Geometry: final body of the model. Coordinates: model frame, mm. Face numbers are marked on the shaded views. Round coordinates to 2 decimals unless told otherwise and drop trailing zeros. Loops run counter-clockwise (first coordinate to the right, second up) from the corner with the lowest first, then second, coordinate; pieces in that order, holes last. Notation, with made-up numbers: (-4, 67.25) - (54, 67.25) arc R18 ccw to (54, 100.25) - close; hole circle Ø6 at (-18, 29.25). An arc over 180 degrees is marked (long way). Return JSON: item names as keys, results as strings. Group by question number.
1. Section C-C on z = 154. Return loops of the section in (x, y), and give its area (3 significant figures).
2. Draft query along X for the marked faces 1 and 2. Return one class per face: +X half, -X half, draft (parallel to the pull), parting line (faces both ways), or undercut.
3. Section D-D on x = 34.5. Return loops of the section in (y, z).
4. Material intervals for probe 1 along Z at (x, y) = (88.9, -0.6); probe 2 along Z at (x, y) = (60, -0.1); probe 3 along Z at (x, y) = (94.5, -0.65), sorted ascending.
5. First-contact query: pin 1 Ø3 at (x, z) = (51.5, 147) entering from +Y. Flat tip, straight axial feed; report the tip coordinate or a pass-through.
6. Section A-A on y = -0.2. Return loops of the section in (x, z).
7. Section B-B on x = 88.9. Return loops of the section in (y, z).
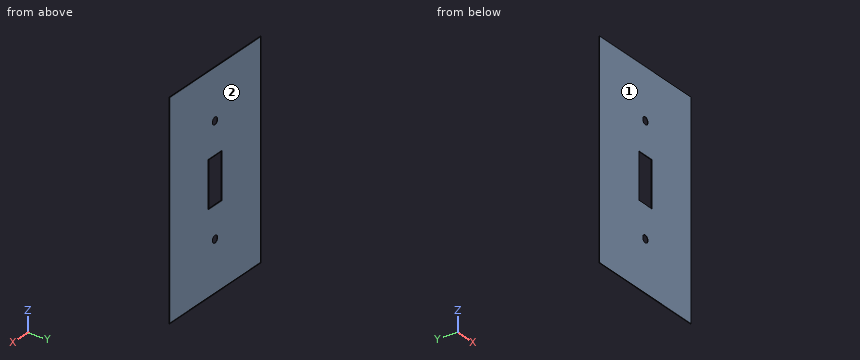
from build123d import *

# Parameters (mm, degrees)
F0_W     = 177.8
F0_H     = 292.1
F1_DEPTH = 1.016
F3_W     = 25.4
F3_H     = 63.5
F4_DEPTH = 25.4
F5_T     = -0.508
F6_R     = 5.08
F7_DEPTH = 25.4
F8_R     = 5.08
F9_DEPTH = 25.4


with BuildPart() as f1:
    # F0 (on Front) → F1 (new body)
    with BuildSketch(Plane.XZ):
        with Locations((88.9, 146.05)):
            Rectangle(F0_W, F0_H)
    extrude(amount=F1_DEPTH)

    # F3 (on face) → F4 (cut)
    with BuildSketch(Plane.XZ.offset(1.016)):
        with Locations((88.9, 146.05)):
            Rectangle(F3_W, F3_H)
    extrude(amount=-F4_DEPTH, mode=Mode.SUBTRACT)

    # F5
    f5_openings = [f1.faces().sort_by_distance(p)[0] for p in [
        (3.41958, 0, 146.05),
    ]]
    offset(amount=F5_T, openings=f5_openings, kind=Kind.INTERSECTION)

    # F6 (on face) → F7 (cut)
    with BuildSketch(Plane.XZ.offset(1.016)):
        with Locations((88.9, 69.85)):
            Circle(F6_R)
    extrude(amount=-F7_DEPTH, mode=Mode.SUBTRACT)

    # F8 (on face) → F9 (cut)
    with BuildSketch(Plane.XZ.offset(1.016)):
        with Locations((88.9, 222.25)):
            Circle(F8_R)
    extrude(amount=-F9_DEPTH, mode=Mode.SUBTRACT)


solid = f1.part
Taken from the geometry:
{
 "1": {"outline": "(0, -1.02) - (76.2, -1.02) - (76.2, 0) - (75.69, 0) - (75.69, -0.51) - (0.51, -0.51) - (0.51, 0) - (0, 0) - close; (101.6, -1.02) - (177.8, -1.02) - (177.8, 0) - (177.29, 0) - (177.29, -0.51) - (102.11, -0.51) - (102.11, 0) - (101.6, 0) - close", "area": "78.5 mm2"},
 "2": {"face 1": "draft", "face 2": "undercut"},
 "3": {"outline": "(-1.02, 0) - (0, 0) - (0, 0.51) - (-0.51, 0.51) - (-0.51, 291.59) - (0, 291.59) - (0, 292.1) - (-1.02, 292.1) - close"},
 "4": {"probe 1": "0 to 64.77, 74.93 to 114.3, 177.8 to 217.17, 227.33 to 292.1", "probe 2": "0 to 0.51, 291.59 to 292.1", "probe 3": "0 to 114.3, 177.8 to 292.1"},
 "5": {"pin 1": "y = -0.51"},
 "6": {"outline": "(0, 0) - (177.8, 0) - (177.8, 292.1) - (0, 292.1) - close; (75.69, 113.79) - (102.11, 113.79) - (102.11, 178.31) - (75.69, 178.31) - close; hole (0.51, 0.51) - (177.29, 0.51) - (177.29, 291.59) - (0.51, 291.59) - close; hole (76.2, 114.3) - (101.6, 114.3) - (101.6, 177.8) - (76.2, 177.8) - close"},
 "7": {"outline": "(-1.02, 0) - (0, 0) - (0, 0.51) - (-0.51, 0.51) - (-0.51, 64.77) - (-1.02, 64.77) - close; (-1.02, 74.93) - (-0.51, 74.93) - (-0.51, 113.79) - (0, 113.79) - (0, 114.3) - (-1.02, 114.3) - close; (-1.02, 177.8) - (0, 177.8) - (0, 178.31) - (-0.51, 178.31) - (-0.51, 217.17) - (-1.02, 217.17) - close; (-1.02, 227.33) - (-0.51, 227.33) - (-0.51, 291.59) - (0, 291.59) - (0, 292.1) - (-1.02, 292.1) - close"}
}
